from build123d import *

# Parameters (mm, degrees)
F6_DEPTH = 40
F7_T     = -2.5


with BuildPart() as f5:
    # F2 (on Top) → F5 section 0
    with BuildSketch(Plane.XY):
        Polygon((-31.8264335891, -18.375), (0, -36.75), (31.8264335891, -18.375), (31.8264335891, 18.375), (0, 36.75), (-31.8264335891, 18.375), align=None)
    # F4 (on offset) → F5 section 1
    with BuildSketch(Plane.XY.offset(25)):
        Polygon((-45.4663336987, -26.25), (0, -52.5), (45.4663336987, -26.25), (45.4663336987, 26.25), (0, 52.5), (-45.4663336987, 26.25), align=None)
    loft()

    # F6 (add): a face of the model
    f6_faces = [f5.faces().sort_by_distance(p)[0] for p in [
        (0, 0, 25),
    ]]
    extrude(f6_faces, amount=F6_DEPTH)

    # F7
    f7_openings = [f5.faces().sort_by_distance(p)[0] for p in [
        (0, 0, 65),
    ]]
    offset(amount=F7_T, openings=f7_openings, kind=Kind.INTERSECTION)


solid = f5.part
Build history of the part. All positions in model axes, mm. A direction names the side the tool comes from. Coordinates: 2 decimals unless noted, no trailing zeros. Order: outer loops, then holes, each group sorted by start corner. A loop starts at its lowest first (then second) coordinate and runs counter-clockwise, first axis right, second up. Notation, with made-up numbers: (-6, 27) - (36, 27) arc R23 cw to (36, 41) - close; hole circle Ø1 at (87, 31). An arc over 180 degrees is marked (long way). Write each question's results on one line, items separated by ' | '. Start each with the question number.
Item 1: Tool access for faces 1 (the face through (-23.05, -39.19, 44.72)), 2 (the face through (-21.78, -37.04, 45.04)): list every direction of +Z, -Z, +X, -X, +Y, -Y with a clear straight run to the whole face (end or side of a thin tool).
Item 2: Mould opens along X. For faces 3 (the face through (23.05, 39.19, 44.72)), 4 (the face through (44, 2, 65)), 5 (the face through (36.743, -0.347, 14.231)) say: released by +X, released by -X, zero draft, split by the parting line, or undercut.
Item 3: Flat gauge pins, fed straight in: pin 1 (1.5 mm diameter, centred on x = -6.5, z = 16, fed in from +Y); pin 2 (5 mm diameter, centred on x = -9, y = 36, fed in from +Z); pin 3 (1 mm diameter, centred on x = 28.5, z = 23, fed in from +Y). Where does each tip first touch, or does it go through?
Item 4: Wall check: probe 1 along X at (y, z) = (1.5, 29.5); probe 2 along Z at (x, y) = (-27, 7.5); probe 3 along Y at (x, z) = (17.5, 44.5). Give the ranges that are in metal, low to high. Write a range as [from, to].
Item 5: Band-saw the part on A-A on z = 31. Write the cut outline in (x, y), and give its area (3 significant figures).
Numbers:
1) face 1: +Z, -Z, -X, -Y | face 2: +Z
2) face 3: released by +X | face 4: zero draft | face 5: undercut
3) pin 1: y = 43.72 | pin 2: z = 16.86 | pin 3: y = 35.21
4) probe 1: [-45.47, -42.97], [42.97, 45.47] | probe 2: [0, 2.5] | probe 3: [-42.4, -39.51], [39.51, 42.4]
5) outline: (-45.47, -26.25) - (0, -52.5) - (45.47, -26.25) - (45.47, 26.25) - (0, 52.5) - (-45.47, 26.25) - close; hole (-42.97, -24.81) - (0, -49.61) - (42.97, -24.81) - (42.97, 24.81) - (0, 49.61) - (-42.97, 24.81) - close | area: 766 mm^2
